For this review, take the finished solid that the model builds, in its own axes (mm). Face numbers are marked on the shaded views. A direction names the side the tool comes from. Round coordinates to 2 decimals unless told otherwise and drop trailing zeros. Order: outer loops, then holes, each group sorted by start corner. A loop starts at its lowest first (then second) coordinate and runs counter-clockwise, first axis right, second up. Notation, with made-up numbers: (10.5, 58) - (30.5, 58) arc R24 cw to (30.5, 86) - close; hole circle Ø11 at (89, 11.5). An arc over 180 degrees is marked (long way). One line per item, written item: value.
```python
from build123d import *

# Parameters (mm, degrees)
F0_W      = 100
F0_H      = 25
F1_DEPTH  = 5
F2_R      = 2.5
F3_DEPTH  = 25
F4_W      = 45.2307462692
F4_H      = 25
F5_DEPTH  = 10
F6_W      = 35.2307462692
F6_H      = 20
F7_DEPTH  = 78
F8_R      = 4.99999
F9_R      = 5.6856472889
F10_DEPTH = 12.5


# Not quite as in the source:
# - a fillet or chamfer is up to 0.001 mm smaller than in the source, because OpenCascade refuses the exact size


with BuildPart() as f1:
    # F0 (on Top) → F1 (new body)
    with BuildSketch(Plane.XY):
        Rectangle(F0_W, F0_H)
    extrude(amount=F1_DEPTH)

    # F2 (on face) → F3 (cut)
    with BuildSketch(Plane.XY.offset(5)):
        with Locations((-37.5, 0)):
            Circle(F2_R)
        with Locations((37.5, 0)):
            Circle(F2_R)
    extrude(amount=-F3_DEPTH, mode=Mode.SUBTRACT)

    # F4 (on face) → F5 (join)
    with BuildSketch(Plane.XY.offset(5)):
        Rectangle(F4_W, F4_H)
    extrude(amount=F5_DEPTH)

    # F6 (on face) → F7 (cut)
    with BuildSketch(Plane.XZ.offset(12.5)):
        Rectangle(F6_W, F6_H)
    extrude(amount=-F7_DEPTH, mode=Mode.SUBTRACT)

    # F8 (radius 5 in the source; OpenCascade refuses exactly that, so slightly less here)
    f8_edges = [f1.edges().sort_by_distance(p)[0] for p in [
        (22.615373, 0, 5),
        (-22.615373, 0, 5),
        (-22.615373, 0, 15),
        (22.615373, 0, 15),
        (50, 0, 5),
        (-50, 0, 5),
        (-17.615373, 0, 10),
        (17.615373, 0, 10),
    ]]
    fillet(f8_edges, radius=F8_R)

    # F9 (on face) → F10 (cut, symmetric)
    with BuildSketch(Plane.XY.offset(5)):
        with Locations((-22.8596497327, 11.807994917)):
            Circle(F9_R)
    extrude(amount=F10_DEPTH, both=True, mode=Mode.SUBTRACT)


solid = f1.part
```
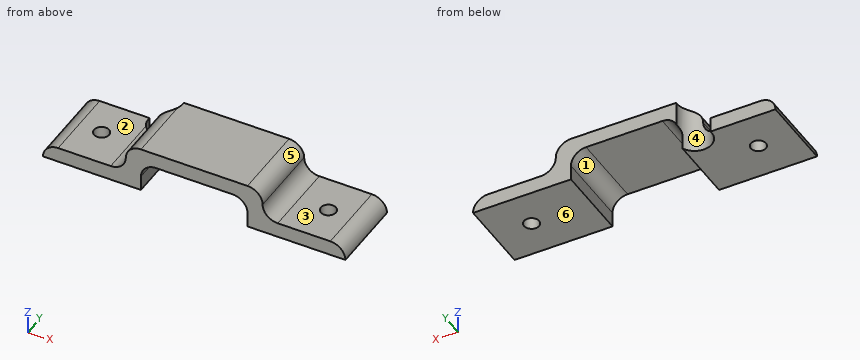
Item 1: Take a section at A-A (x = 37.5). Write out the cut boundary in (y, z).
Returned:
outline: (-12.5, 0) - (-2.5, 0) - (-2.5, 5) - (-12.5, 5) - close; (2.5, 0) - (12.5, 0) - (12.5, 5) - (2.5, 5) - close
Item 2: Wall thickness on line 1 (Y direction, x = 37.5, z = 2); line 2 (X direction, y = 7.75, z = 2.25); line 3 (X direction, y = -4, z = 8.5): over which ranges is each line inside the solid? List them lowest first.
Returned:
line 1: -12.5 to -2.5, 2.5 to 12.5
line 2: -49.47 to -26.84, -18.88 to -17.62, 17.62 to 49.47
line 3: -22.85 to -16.19, 16.19 to 22.85
Item 3: The part is to be moulded in two halves that separate along X. For the marked faces 4, 5 and 6, say which applies: +X half, -X half, draft (parallel to the pull), parting line (faces both ways), or undercut.
Returned:
face 4: undercut
face 5: +X half
face 6: draft
Item 4: Machinability: for the marked faces 1, 2 and 3, which of the approach directions +Z, -Z, +X, -X, +Y, -Y give a long, thin tool a straight path to every point of the face, cutting with its end or side? Answer none if there is none.
Returned:
face 1: -Z, +Y, -Y
face 2: +Z, -X, +Y, -Y
face 3: +Z, +X, +Y, -Y
Item 5: For P1, Ø6.5, axis at x = 37.5, y = 0, coming from the +Z side; P2, Ø5, axis at y = 7, z = 12, coming from the +X side; P3, Ø4, axis at y = 1.5, z = 9, coming from the +X side, all flat-tipped, find the tip position at first contact; note any pin that passes through.
Returned:
P1: z = 5
P2: x = 22.64
P3: x = 23.62
Item 6: Take a section at B-B (z = 3.5). Write out the cut boundary in (x, y).
Returned:
outline: (-48.57, -12.5) - (-17.62, -12.5) - (-17.62, 9.61) arc R5.69 cw to (-28.5, 12.5) - (-48.57, 12.5) - close; (17.62, -12.5) - (48.57, -12.5) - (48.57, 12.5) - (17.62, 12.5) - close; hole circle Ø5 at (-37.5, 0); hole circle Ø5 at (37.5, 0)
Item 7: Take a section at D-D (x = 15.5). Write out the cut boundary in (y, z), plus the area to 3 significant figures.
Returned:
outline: (-12.5, 9.08) - (12.5, 9.08) - (12.5, 15) - (-12.5, 15) - close
area: 148 mm^2
